Can you work these out from the drawing? Everything is in mm from the part's minimum corner. Coordinates: 2 decimals unless noted, no trailing zeros. Write each loop counter-clockwise with the first axis right and the second up, starting at its lowest first coordinate (ties: lowest second). Pieces come first, ordered by that corner, then holes. Notation, with made-up numbers: (58, -16) -> (106, -16) arc R33 cw to (106, 19) -> close; hole circle Ø1 at (-7.5, 20.5). An arc over 180 degrees is marked (long way). Use a Markdown table: item, result. Add a question column.
Item 1: Imagine slicing it at D-D, the plane x = 15. Write out the boundary of the cut face in (y, z).
Item 2: Imagine slicing it at C-C, the plane z = 1.5. Write out the boundary of the cut face in (x, y), and give its area (3 significant figures).
Item 3: If I drill on line 1 along Y through (x, z) = (3.75, 1.7); line 2 along Y through (x, z) = (27, 2.45), over which ranges is the centre line in solid material (lowest first)? Write a range as from..to.
Item 4: Imagine slicing it at B-B, the plane y = 30. Write out the boundary of the cut face in (x, z).
Item 5: Imagine slicing it at A-A, the plane x = 3.75. Write out the boundary of the cut face in (y, z), and give its area (3 significant figures).
Item 6: Will this pin go through, and if not, where does the flat tip stop? pin 1 Ø2 at (x, y) = (26.25, 56.25) entering from -Z.
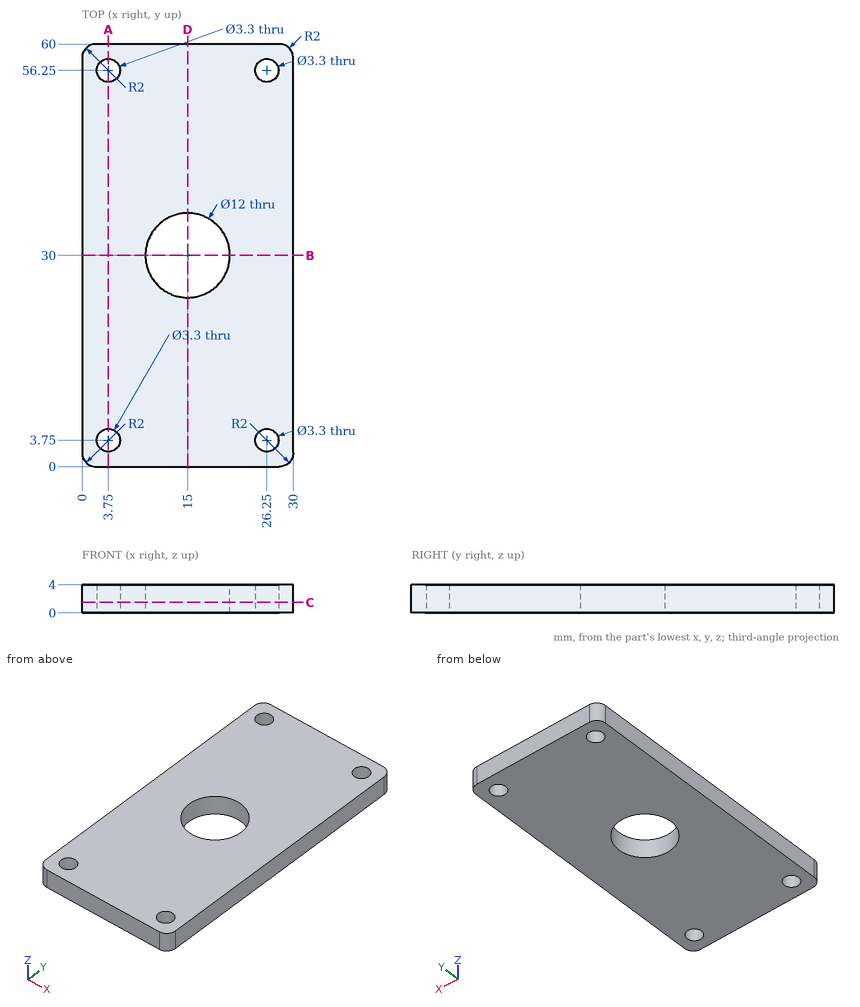
Ans:
| question | item | result |
|---|---|---|
| 1 | outline | (0, 0) -> (24, 0) -> (24, 4) -> (0, 4) -> close; (36, 0) -> (60, 0) -> (60, 4) -> (36, 4) -> close |
| 2 | outline | (0, 2) arc R2 ccw to (2, 0) -> (28, 0) arc R2 ccw to (30, 2) -> (30, 58) arc R2 ccw to (28, 60) -> (2, 60) arc R2 ccw to (0, 58) -> close; hole circle Ø3.3 at (3.75, 3.75); hole circle Ø3.3 at (3.75, 56.25); hole circle Ø12 at (15, 30); hole circle Ø3.3 at (26.25, 3.75); hole circle Ø3.3 at (26.25, 56.25) |
| 2 | area | 1,650 mm^2 |
| 3 | line 1 | y = 0..2.1, 5.4..54.6, 57.9..60 |
| 3 | line 2 | y = 0..2.28, 5.22..54.78, 57.72..60 |
| 4 | outline | (0, 0) -> (9, 0) -> (9, 4) -> (0, 4) -> close; (21, 0) -> (30, 0) -> (30, 4) -> (21, 4) -> close |
| 5 | outline | (0, 0) -> (2.1, 0) -> (2.1, 4) -> (0, 4) -> close; (5.4, 0) -> (54.6, 0) -> (54.6, 4) -> (5.4, 4) -> close; (57.9, 0) -> (60, 0) -> (60, 4) -> (57.9, 4) -> close |
| 5 | area | 214 mm^2 |
| 6 | pin 1 | passes through |
